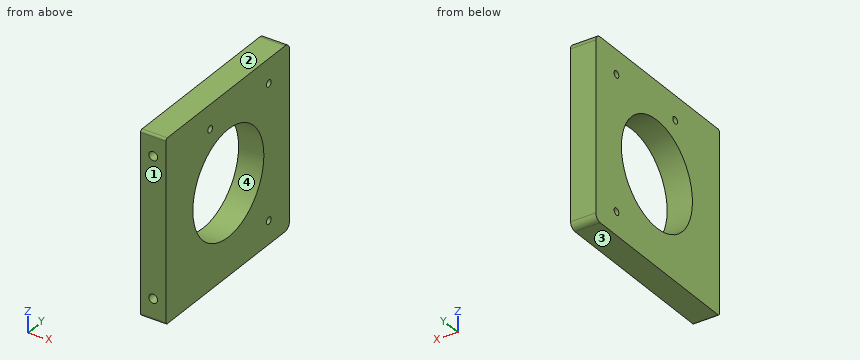
from build123d import *

# Parameters (mm, degrees)
SKETCH1_W           = 40
SKETCH1_H           = 86
BOSS_EXTRUDE1_DEPTH = 12
SKETCH2_W           = 12
SKETCH2_H           = 86
BOSS_EXTRUDE2_DEPTH = 87
SKETCH3_R           = 3
CUT_EXTRUDE1_DEPTH  = 13
SKETCH5_R           = 1.65
CUT_EXTRUDE3_DEPTH  = 13
FILLET1_R           = 3
SKETCH6_R           = 25
CUT_EXTRUDE4_DEPTH  = 13
SKETCH7_W           = 40
SKETCH7_H           = 12
CUT_EXTRUDE5_DEPTH  = 87
SKETCH8_R           = 2.1
CUT_EXTRUDE6_DEPTH  = 12
FILLET2_R           = 1


with BuildPart() as part:
    # Sketch1 → Boss-Extrude1 (new body)
    with BuildSketch(Plane(origin=(0, 0, 0), x_dir=(1, 0, 0), z_dir=(0, 1, 0))):
        with Locations((20, -43)):
            Rectangle(SKETCH1_W, SKETCH1_H)
    extrude(amount=BOSS_EXTRUDE1_DEPTH)

    # Sketch2 → Boss-Extrude2 (add)
    with BuildSketch(Plane(origin=(0, 12, 0), x_dir=(1, 0, 0), z_dir=(0, 1, 0))):
        with Locations((34, -43)):
            Rectangle(SKETCH2_W, SKETCH2_H)
    extrude(amount=BOSS_EXTRUDE2_DEPTH)

    # Sketch3 → Cut-Extrude1 (cut, through all)
    with BuildSketch(Plane(origin=(0, 12, 0), x_dir=(1, 0, 0), z_dir=(0, 1, 0))):
        with Locations((14, -8.4)):
            Circle(SKETCH3_R)
        with Locations((14, -77.6)):
            Circle(SKETCH3_R)
    extrude(amount=-CUT_EXTRUDE1_DEPTH, mode=Mode.SUBTRACT)

    # Sketch5 → Cut-Extrude3 (cut, through all)
    with BuildSketch(Plane.ZY.offset(-28)):
        with Locations((74.5, 84.5)):
            Circle(SKETCH5_R)
        with Locations((74.5, 43.2)):
            Circle(SKETCH5_R)
        with Locations((11, 84.5)):
            Circle(SKETCH5_R)
    extrude(amount=-CUT_EXTRUDE3_DEPTH, mode=Mode.SUBTRACT)

    # Fillet1
    fillet1_edges = [part.edges().sort_by_distance(p)[0] for p in [
        (34, 99, 0),
        (34, 99, 86),
    ]]
    fillet(fillet1_edges, radius=FILLET1_R)

    # Sketch6 → Cut-Extrude4 (cut, through all)
    with BuildSketch(Plane.ZY.offset(-28)):
        with Locations((43, 56)):
            Circle(SKETCH6_R)
    extrude(amount=-CUT_EXTRUDE4_DEPTH, mode=Mode.SUBTRACT)

    # Sketch7 → Cut-Extrude5 (cut, through all)
    with BuildSketch(Plane.XY.offset(86)):
        with Locations((20, 6)):
            Rectangle(SKETCH7_W, SKETCH7_H)
    extrude(amount=-CUT_EXTRUDE5_DEPTH, mode=Mode.SUBTRACT)

    # Sketch8 → Cut-Extrude6 (cut)
    with BuildSketch(Plane.XZ.offset(-12)):
        with Locations((34, 76)):
            Circle(SKETCH8_R)
        with Locations((34, 10)):
            Circle(SKETCH8_R)
    extrude(amount=-CUT_EXTRUDE6_DEPTH, mode=Mode.SUBTRACT)

    # Fillet2
    fillet2_edges = [part.edges().sort_by_distance(p)[0] for p in [
        (34, 12, 0),
        (34, 12, 86),
    ]]
    fillet(fillet2_edges, radius=FILLET2_R)


solid = part.part
Design review of the part built by this model. Coordinates are the model's own, in mm. Face numbers are marked on the shaded views. Give positions to 0.01 mm unless a question says otherwise; leave off trailing zeros. Order: outer loops, then holes, each group sorted by start corner. A loop starts at its lowest first (then second) coordinate and runs counter-clockwise, first axis right, second up. Notation, with made-up numbers: (25, 33) - (78, 33) arc R26 ccw to (78, 71) - close; hole circle Ø9 at (14, -24). An arc over 180 degrees is marked (long way). Use CSV: the item, a comma, the result in double quotes. Start each with the question number.
Q1. Take a section at B-B (z = 42). State the section outline as (x, y) points.
Q2. Take a section at D-D (y = 57). State the section outline as (x, z) points.
Q3. Take a section at C-C (x = 29.5). State the section outline as (y, z) points.
Q4. For line 1 (Y direction, x = 31.25, z = 74.5); line 2 (Z direction, x = 32.25, y = 84.5); line 3 (Y direction, x = 30.25, z = 22.5), list the stretches that pass through material, from the lowest coordinate up.
Q5. Draft analysis for pull direction Z (two halves, no side actions). For the marked faces 1, 2, 3 and 4, state which applies: pulls with the +Z half, pulls with the -Z half, needs draft (parallel to the pull), parting line crosses it, or undercut.
Q6. For P1, Ø2.5, axis at y = 84.5, z = 11, coming from the +X side; P2, Ø3.5, axis at x = 34, z = 10, coming from the -Y side, all flat-tipped, find the tip position at first contact; note any pin that passes through.
Q7. Take a section at A-A (y = 84.5). State the section outline as (x, z) points.
Calculated:
1,outline,"(28, 12) - (40, 12) - (40, 31.02) - (28, 31.02) - close; (28, 80.98) - (40, 80.98) - (40, 99) - (28, 99) - close"
2,outline,"(28, 0) - (40, 0) - (40, 18.02) - (28, 18.02) - close; (28, 67.98) - (40, 67.98) - (40, 86) - (28, 86) - close"
3,outline,"(12, 1) arc R1 ccw to (13, 0) - (96, 0) arc R3 ccw to (99, 3) - (99, 83) arc R3 ccw to (96, 86) - (13, 86) arc R1 ccw to (12, 85) - close; hole circle Ø50 at (56, 43); hole circle Ø3.3 at (43.2, 74.5); hole circle Ø3.3 at (84.5, 11); hole circle Ø3.3 at (84.5, 74.5)"
4,line 1,"y = 12 to 41.55, 44.85 to 82.85, 86.15 to 99"
4,line 2,"z = 0 to 9.35, 12.65 to 72.85, 76.15 to 86"
4,line 3,"y = 12 to 41.69, 70.31 to 99"
5,face 1,"needs draft"
5,face 2,"pulls with the +Z half"
5,face 3,"pulls with the -Z half"
5,face 4,"undercut"
6,P1,"passes through"
6,P2,"stops at y = 24"
7,outline,"(28, 0) - (40, 0) - (40, 9.35) - (28, 9.35) - close; (28, 12.65) - (40, 12.65) - (40, 72.85) - (28, 72.85) - close; (28, 76.15) - (40, 76.15) - (40, 86) - (28, 86) - close"
